CAD build for the part. Positions are in the model's coordinates, mm. A direction names the side the tool comes from. Round coordinates to 2 decimals unless told otherwise and drop trailing zeros. Loops run counter-clockwise (first coordinate to the right, second up) from the corner with the lowest first, then second, coordinate; pieces in that order, holes last. Notation, with made-up numbers: (17, -8) - (27, -8) arc R32 cw to (27, 19) - close; hole circle Ø11 at (18, -37.75). An arc over 180 degrees is marked (long way). One line per question, with ' | ' between items.
```python
from build123d import *

# Parameters (mm, degrees)
BOSS_EXTRUDE1_DEPTH      = 10
BOSS_EXTRUDE2_DEPTH      = 25
SKETCH11_R               = 1
CUT_EXTRUDE9_DEPTH       = 37.472090445
CUT_EXTRUDE16_DEPTH      = 14.1
CUT_EXTRUDE16_DEPTH_BACK = 14.1


with BuildPart() as part:
    # Sketch1 → Boss-Extrude1 (new body)
    with BuildSketch(Plane.XY):
        with BuildLine():
            Line((10, 0), (-10, 0))
            Line((-10, 0), (-10, 25))
            ThreePointArc((-10, 25), (0, 35), (10, 25))
            Line((10, 25), (10, 0))
        make_face()
    extrude(amount=BOSS_EXTRUDE1_DEPTH)

    # Sketch16 → Boss-Extrude2 (add)
    with BuildSketch(Plane.XZ):
        with BuildLine():
            Line((-10, 0), (-10, 10))
            ThreePointArc((-10, 10), (-11.472090345, 5), (-10, 0))
        make_face()
        with BuildLine():
            Line((10, 0), (10, 10))
            ThreePointArc((10, 10), (11.472090345, 5), (10, 0))
        make_face()
    extrude(amount=-BOSS_EXTRUDE2_DEPTH)

    # Sketch18 → Revolve1 (revolve)
    with BuildSketch(Plane(origin=(0, 25, 0), x_dir=(1, 0, 0), z_dir=(0, 1, 0))):
        with BuildLine():
            Line((10, 0), (10, -10))
            ThreePointArc((10, -10), (11.472090345, -5), (10, 0))
        make_face()
    revolve(axis=Axis((0, 25, 0), (0, 0, 1)))

    # Sketch11 → Cut-Extrude9 (cut, through all)
    with BuildSketch(Plane.XZ):
        with Locations((4, 2.295920755)):
            Circle(SKETCH11_R)
        with Locations((-4, 2.295920755)):
            Circle(SKETCH11_R)
    extrude(amount=-CUT_EXTRUDE9_DEPTH, mode=Mode.SUBTRACT)

    # Sketch14 → Cut-Extrude16 (cut, two sides)
    with BuildSketch(Plane.ZY) as cut_extrude16_sk:
        with BuildLine():
            Line((4.95, 1.181346652), (4.95, 0))
            Line((4.95, 0), (7.05, 0))
            Line((7.05, 0), (7.05, 1.181346652))
            ThreePointArc((7.05, 1.181346652), (6, 5.1), (4.95, 1.181346652))
        make_face()
    extrude(amount=CUT_EXTRUDE16_DEPTH, mode=Mode.SUBTRACT)
    extrude(cut_extrude16_sk.sketch, amount=-CUT_EXTRUDE16_DEPTH_BACK, mode=Mode.SUBTRACT)


solid = part.part
```
(1) Tool access for faces 4 (the face through (0, 1, 4.95)), 5 (the face through (0, 18, 10)): list every direction of +Z, -Z, +X, -X, +Y, -Y with a clear straight run to the whole face (end or side of a thin tool).
Results found:
face 4: +X, -X, -Y | face 5: +Z, +X, -X, +Y, -Y
(2) Cut at B-B, the plane y = 15. Write the cut outline in (x, z), then the cut area to 3 significant figures.
Results found:
outline: (-10, 0) - (10, 0) arc R9.23 ccw to (10, 10) - (-10, 10) arc R9.23 ccw to start; hole circle Ø2 at (-4, 2.3); hole circle Ø2 at (4, 2.3) | area: 214 mm²
(3) Cut at A-A, the plane y = 3. Write the cut outline in (x, z).
Results found:
outline: (-11.41, 3.9) arc R9.23 ccw to (-10, 0) - (10, 0) arc R9.23 ccw to (11.41, 3.9) - close; (-10.94, 8.1) - (10.94, 8.1) arc R9.23 ccw to (10, 10) - (-10, 10) arc R9.23 ccw to start; hole circle Ø2 at (-4, 2.3); hole circle Ø2 at (4, 2.3)
(4) Two-plate mould, pull along X, no slides. Class faces 1 (the face through (3, 17.6, 2.3)), 2 (the face through (11.47, 12.32, 5.07)), 3 (the face through (0.16, 5.1, 6.08)): released by +X, released by -X, zero draft, split by the parting line, or undercut.
Results found:
face 1: undercut | face 2: released by +X | face 3: zero draft
(5) Drop a flat-ended pin along its axis: P1, Ø2, axis at x = -1.5, z = 3, coming from the +Y side. Give the stop position or say it passes through.
Results found:
P1: stops at y = 36.36
(6) Probe L1, parallel to Z at x = 4, y = 28.5; L2, parallel to Z at x = 5.5, y = 3; L3, parallel to X at y = 27, z = 1.5. List the from-to ranges inside material, lowest first.
Results found:
L1: z = 0 to 1.3, 3.3 to 10 | L2: z = 0 to 3.9, 8.1 to 10 | L3: x = -10.6 to -4.61, -3.39 to 3.39, 4.61 to 10.6
